Geometry check sheet. Reference: drawing and pictorial views, mm from the part's lowest x, y, z. A direction names the side the tool comes from. Coordinates: 2 decimals unless noted, no trailing zeros. Write each loop counter-clockwise with the first axis right and the second up, starting at its lowest first coordinate (ties: lowest second). Pieces come first, ordered by that corner, then holes. Notation, with made-up numbers: (46, -4.5) -> (87, -4.5) arc R28 cw to (87, 16.5) -> close; hole circle Ø10 at (55.5, 3.5). An arc over 180 degrees is marked (long way). Answer in a Markdown table with one row per item.
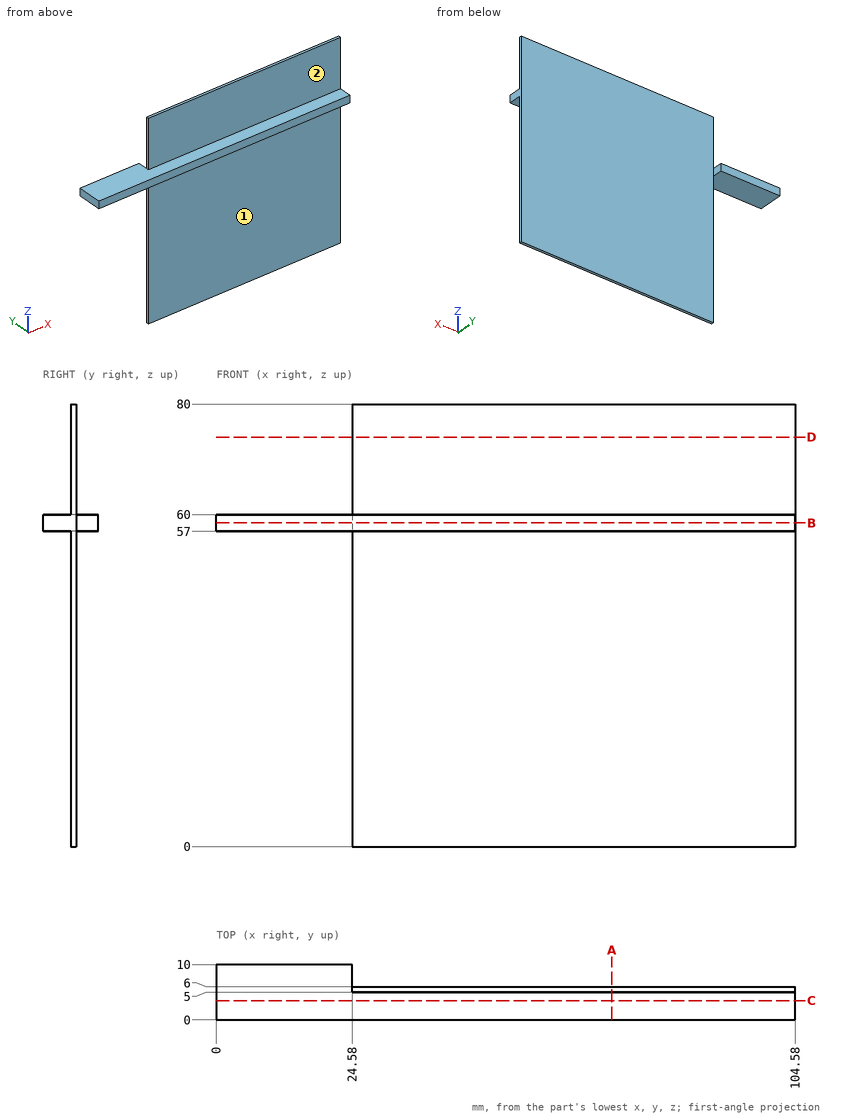
1. Tool access check on the marked faces 1 and 2. Record the directions out of +Z, -Z, +X, -X, +Y, -Y that give a thin tool (end or side, any length) a straight path to the whole face; none if there is none.
Geometry says:
| item | result |
|---|---|
| face 1 | -Z, +X, -X, -Y |
| face 2 | +Z, +X, -X, -Y |
2. Section check C-C, the plane y = 3.5. Record the boundary of the cut face in (x, z), plus the area to 3 significant figures.
Geometry says:
| item | result |
|---|---|
| outline | (0, 57) -> (104.58, 57) -> (104.58, 60) -> (0, 60) -> close |
| area | 314 mm^2 |
3. Section check A-A, the plane x = 71.5. Record the boundary of the cut face in (y, z), plus the area to 3 significant figures.
Geometry says:
| item | result |
|---|---|
| outline | (0, 57) -> (5, 57) -> (5, 0) -> (6, 0) -> (6, 80) -> (5, 80) -> (5, 60) -> (0, 60) -> close |
| area | 95.0 mm^2 |
4. Depth check by flat-ended pin: P1, Ø4, axis at x = 13, y = 5, coming from the -Z side; P2, Ø0.8, axis at y = 5.5, z = 75, coming from the -X side; P3, Ø24, axis at x = 76, z = 55, coming from the +Y side. Enter the tip coordinate at first touch or a pass-through.
Geometry says:
| item | result |
|---|---|
| P1 | z = 57 |
| P2 | x = 24.58 |
| P3 | y = 6 |
5. Thickness scan on line 1 (Z direction, x = 22.5, y = 7); line 2 (Y direction, x = 41.5, z = 76.5); line 3 (X direction, y = 5.75, z = 51). Record the ranges inside material, lowest first. Write a range as from..to.
Geometry says:
| item | result |
|---|---|
| line 1 | 57..60 |
| line 2 | 5..6 |
| line 3 | 24.58..104.58 |
6. Section check B-B, the plane z = 58.5. Record the boundary of the cut face in (x, y).
Geometry says:
| item | result |
|---|---|
| outline | (0, 0) -> (104.58, 0) -> (104.58, 6) -> (24.58, 6) -> (24.58, 10) -> (0, 10) -> close |
7. Section check D-D, the plane z = 74. Record the boundary of the cut face in (x, y).
Geometry says:
| item | result |
|---|---|
| outline | (24.58, 5) -> (104.58, 5) -> (104.58, 6) -> (24.58, 6) -> close |
